The drawing under review shows one solid part. Ordinate dimensions are in mm from its lowest x, y, z. Give positions to 0.01 mm unless a question says otherwise; leave off trailing zeros. Loops run counter-clockwise (first coordinate to the right, second up) from the corner with the lowest first, then second, coordinate; pieces in that order, holes last. Notation, with made-up numbers: (22, -23.5) -> (28, -23.5) arc R19 cw to (28, -4.5) -> close; hole circle Ø8 at (50, 66.5). An arc over 180 degrees is marked (long way). Answer in a Markdown table with one row per item. Add a question column.
(1) Consider section C-C on z = 4.75. Write out the cut boundary in (x, y).
(2) For pin 1 (5 mm diameter, centred on x = 46.5, z = 14, fed in from +Y); pin 2 (4.5 mm diameter, centred on x = 55.98, y = 34.02, fed in from +Z); pin 3 (2 mm diameter, centred on x = 41, y = 37.5, fed in from -Z); pin 4 (10 mm diameter, centred on y = 37.5, z = 5, fed in from -X), all flat-tipped, find the tip position at first contact; note any pin that passes through.
(3) Consider section A-A on x = 45. Write out the cut boundary in (y, z), then the cut area to 3 significant figures.
(4) For line 1 (Z direction, x = 69, y = 65.5); line 2 (X direction, y = 37, z = 3.5); line 3 (X direction, y = 67, z = 15) (1 decimal), list the stretches that pass through material, from the lowest coordinate up.
(5) Consider section D-D on x = 17.5. Write out the cut boundary in (y, z).
(6) Draft analysis for pull direction Y (two halves, no side actions). For the marked faces 1, 2 and 3, state which applies: +Y half, -Y half, draft (parallel to the pull), parting line (faces both ways), or undercut.
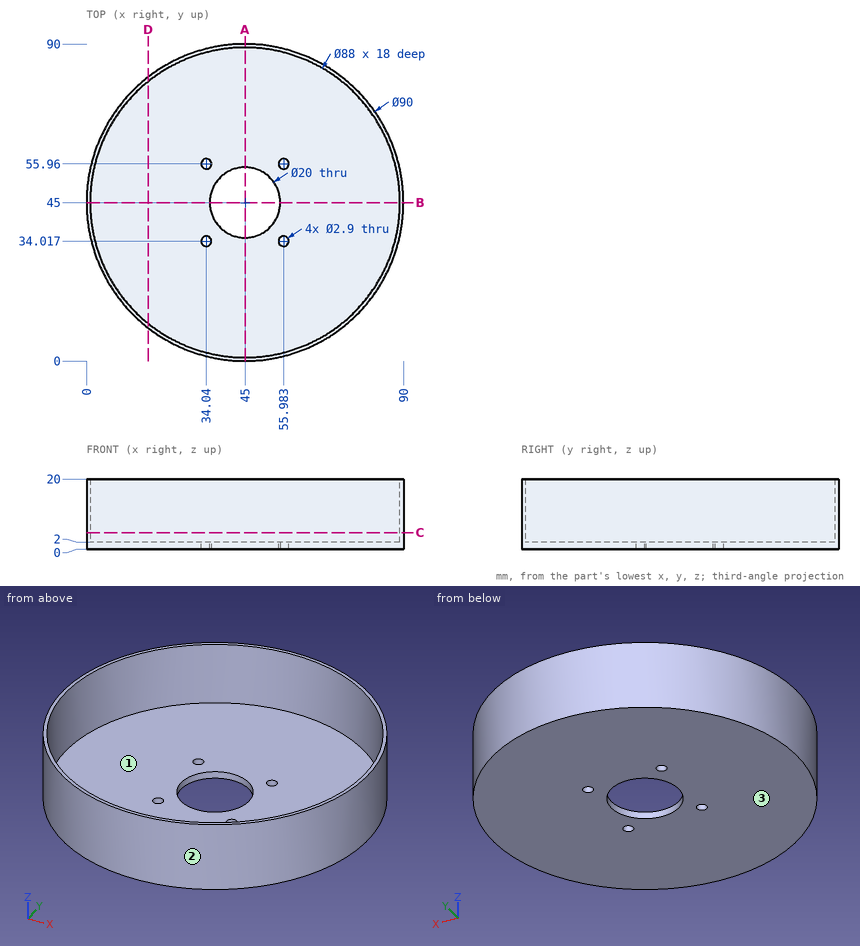
Values follow:
| question | item | result |
|---|---|---|
| 1 | outline | circle Ø90 at (45, 45); hole circle Ø88 at (45, 45) |
| 2 | pin 1 | y = 90 |
| 2 | pin 2 | z = 2 |
| 2 | pin 3 | through |
| 2 | pin 4 | x = 0.07 |
| 3 | outline | (0, 0) -> (35, 0) -> (35, 2) -> (1, 2) -> (1, 20) -> (0, 20) -> close; (55, 0) -> (90, 0) -> (90, 20) -> (89, 20) -> (89, 2) -> (55, 2) -> close |
| 3 | area | 176 mm2 |
| 4 | line 1 | 0 to 2 |
| 4 | line 2 | 0.72 to 1.73, 88.27 to 89.28 |
| 4 | line 3 | 5.7 to 6.9, 83.1 to 84.3 |
| 5 | outline | (9.38, 0) -> (80.62, 0) -> (80.62, 20) -> (79.35, 20) -> (79.35, 2) -> (10.65, 2) -> (10.65, 20) -> (9.38, 20) -> close |
| 6 | face 1 | undercut |
| 6 | face 2 | parting line |
| 6 | face 3 | draft |
